Work out the finished part from the listing and answer in its coordinate system (mm). Give positions to 0.01 mm unless a question says otherwise; leave off trailing zeros. Loops run counter-clockwise (first coordinate to the right, second up) from the corner with the lowest first, then second, coordinate; pieces in that order, holes last.
```python
from build123d import *

# Parameters (mm, degrees)
SKETCH1_R           = 1.75
SKETCH1_R_2         = 1.25
BOSS_EXTRUDE1_DEPTH = 3
FILLET1_R           = 10


with BuildPart() as part:
    # Sketch1 → Boss-Extrude1 (new body)
    with BuildSketch(Plane.XY):
        with BuildLine():
            Line((-90.476878828, 136.710551041), (-11.976878828, 0.744562647))
            ThreePointArc((-11.976878828, 0.744562647), (6, -10.392304845), (5.343629247, 10.744562647))
            Line((5.343629247, 10.744562647), (-73.156370753, 146.710551041))
            Line((-73.156370753, 146.710551041), (-90.476878828, 136.710551041))
        make_face()
        with Locations((-76.81662479, 133.050297003)):
            Circle(SKETCH1_R, mode=Mode.SUBTRACT)
        with Locations((8, 0)):
            Circle(SKETCH1_R_2, mode=Mode.SUBTRACT)
        with Locations((-4, -6.92820323)):
            Circle(SKETCH1_R_2, mode=Mode.SUBTRACT)
        with Locations((-8, 0)):
            Circle(SKETCH1_R_2, mode=Mode.SUBTRACT)
        with Locations((-4, 6.92820323)):
            Circle(SKETCH1_R_2, mode=Mode.SUBTRACT)
        with Locations((4, 6.92820323)):
            Circle(SKETCH1_R_2, mode=Mode.SUBTRACT)
    extrude(amount=BOSS_EXTRUDE1_DEPTH)

    # Fillet1
    fillet1_edges = [part.edges().sort_by_distance(p)[0] for p in [
        (-11.976878828, 0.744562647, 1.5),
        (5.343629247, 10.744562647, 1.5),
        (-90.476878828, 136.710551041, 1.5),
        (-73.156370753, 146.710551041, 1.5),
    ]]
    fillet(fillet1_edges, radius=FILLET1_R - 0.0001)  # a hair under: the kernel refuses the full size


solid = part.part
```
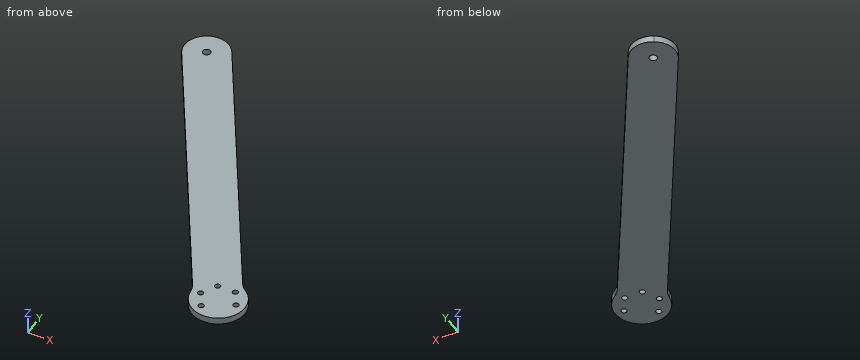
Q1. Given pin 1 (1.5 mm diameter, centred on x = -17.5, z = 1.5, fed in from +Y), flat-ended and moving along its own axis, determine where the tip first touches the part or whether it passes through.
Q2. Section B-B on x = 0 is taken. Give the vertices of the cut face in (y, z), plus the area to 3 significant figures.
Q3. Section C-C on y = 88.5 is taken. Give the vertices of the cut face in (x, z), plus the area to 3 significant figures.
Q4. Consider line 1 along Y through (x, z) = (-4, 1); line 2 along X through (y, z) = (113.5, 1.35); line 3 along X through (y, z) = (35, 2.75). Determine where each line is inside the solid, lowest interval first.
Q5. Section A-A on z = 1 is taken. State how many separate pieces and enclosed holes the cut face has, plus the area to 3 significant figures.
Check result:
1. pin 1: stops at y = 51.61
2. outline: (-12, 0) - (20, 0) - (20, 3) - (-12, 3) - close
2. area: 96.0 mm2
3. outline: (-62.64, 0) - (-39.55, 0) - (-39.55, 3) - (-62.64, 3) - close
3. area: 69.3 mm2
4. line 1: y = -11.31 to -8.18, -5.68 to 5.68, 8.18 to 26.93
4. line 2: x = -77.08 to -53.98
4. line 3: x = -31.75 to -8.66
5. separate pieces: 1
5. enclosed holes: 6
5. area: 3,440 mm2
